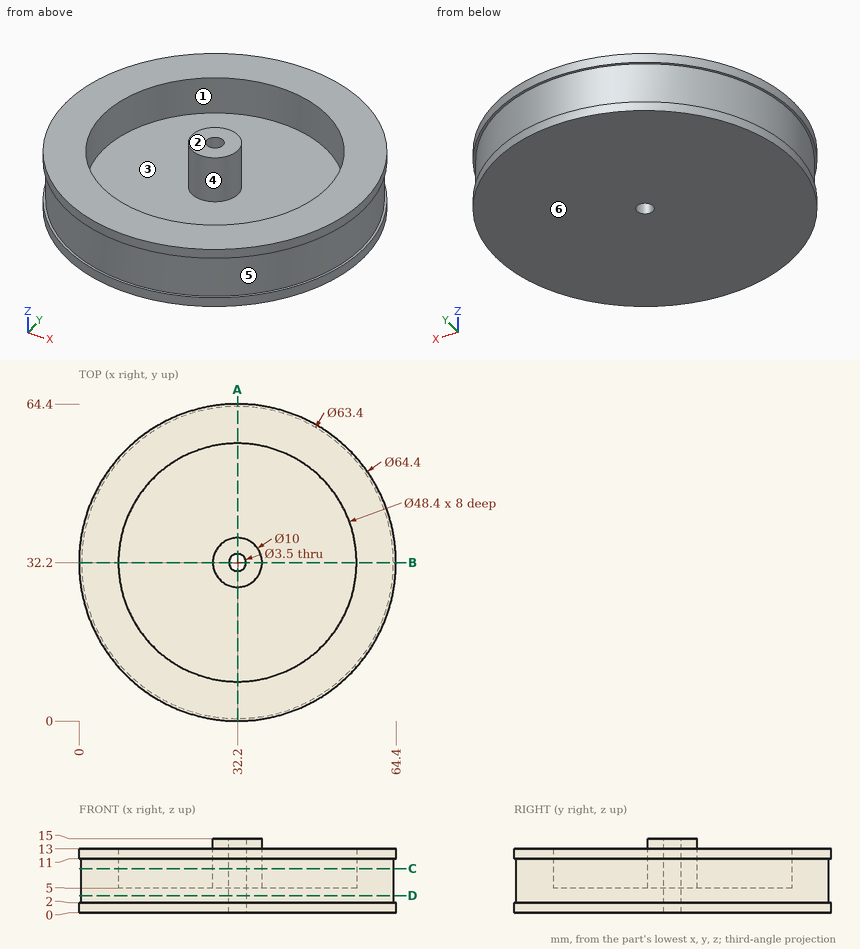
Could you check a few things on this drawing? It's one solid part, dimensions in mm from its lowest x, y, z. A direction names the side the tool comes from. Coordinates: 2 decimals unless noted, no trailing zeros. Write each loop counter-clockwise with the first axis right and the second up, starting at its lowest first coordinate (ties: lowest second). Pieces come first, ordered by that corner, then holes. Notation, with made-up numbers: (-25.75, 32.25) - (-17.75, 32.25) arc R27 cw to (-17.75, 61.25) - close; hole circle Ø4 at (33, 34). An arc over 180 degrees is marked (long way). Return JSON: item names as keys, results as strings. Group by question number.
Item 1: If we section it at D-D (z = 3.5): Write out the boundary of the cut face in (x, y), then the cut area to 3 significant figures.
Item 2: If we section it at A-A (x = 32.2): Write out the boundary of the cut face in (y, z).
Item 3: We'd pull the mould along Z, two halves only. Please class the marked faces 3, 4, 5 and 6: pulls with the +Z half, pulls with the -Z half, needs draft (parallel to the pull), parting line crosses it, or undercut.
Item 4: I'm going to push flat-ended pins straight in: pin 1 Ø8 at (x, y) = (42.5, 31) entering from +Z; pin 2 Ø1.5 at (y, z) = (35, 10) entering from +X; pin 3 Ø1.5 at (x, z) = (27, 12.5) entering from +Y; pin 4 Ø2 at (x, y) = (32.2, 32.2) entering from -Z. Where does each tip first touch, or does it pass through?
Item 5: Which directions (+Z, -Z, +X, -X, +Y, -Y) give clear straight access to the entire face, cutting with the end or side of a thin tool? Please do the marked faces 1 and 2.
Item 6: Please list where these lines run through material, in increasing order: probe 1 along Y at (x, z) = (32.2, 5.25); probe 2 along Z at (x, y) = (52, 56.5); probe 3 along Z at (x, y) = (30, 49.5).
Item 7: If we section it at C-C (z = 9): Write out the boundary of the cut face in (x, y), then the cut area to 3 significant figures.
Return value:
{
 "1": {"outline": "circle Ø63.4 at (32.2, 32.2); hole circle Ø3.5 at (32.2, 32.2)", "area": "3,150 mm^2"},
 "2": {"outline": "(0, 0) - (30.45, 0) - (30.45, 15) - (27.2, 15) - (27.2, 5) - (8, 5) - (8, 13) - (0, 13) - (0, 11) - (0.5, 11) - (0.5, 2) - (0, 2) - close; (33.95, 0) - (64.4, 0) - (64.4, 2) - (63.9, 2) - (63.9, 11) - (64.4, 11) - (64.4, 13) - (56.4, 13) - (56.4, 5) - (37.2, 5) - (37.2, 15) - (33.95, 15) - close"},
 "3": {"face 3": "pulls with the +Z half", "face 4": "needs draft", "face 5": "undercut", "face 6": "pulls with the -Z half"},
 "4": {"pin 1": "stops at z = 5", "pin 2": "stops at x = 63.83", "pin 3": "stops at y = 64.09", "pin 4": "passes through"},
 "5": {"face 1": "+Z", "face 2": "+Z, +X, -X, +Y, -Y"},
 "6": {"probe 1": "y = 0.5 to 8, 27.2 to 30.45, 33.95 to 37.2, 56.4 to 63.9", "probe 2": "z = 0 to 13", "probe 3": "z = 0 to 5"},
 "7": {"outline": "circle Ø63.4 at (32.2, 32.2); circle Ø10 at (32.2, 32.2); hole circle Ø48.4 at (32.2, 32.2); hole circle Ø3.5 at (32.2, 32.2)", "area": "1,390 mm^2"}
}
